Read the model definition and answer for the solid it produces. Units are mm, in the model's axes. Face numbers are marked on the shaded views. Coordinates: 2 decimals unless noted, no trailing zeros. Write each loop counter-clockwise with the first axis right and the second up, starting at its lowest first coordinate (ties: lowest second). Pieces come first, ordered by that corner, then holes. Notation, with made-up numbers: (86, 58) -> (111, 58) arc R27 cw to (111, 74) -> close; hole circle Ø6 at (61.25, -39.5). An arc over 180 degrees is marked (long way). One line per item, written item: value. Start each with the question number.
from build123d import *

# Parameters (mm, degrees)
ESQUISSE1_W         = 41
ESQUISSE1_H         = 30.4
BOSS_EXTRU_1_DEPTH  = 2
ESQUISSE3_R         = 3
BOSS_EXTRU_2_DEPTH  = 2
ESQUISSE4_W         = 15
ESQUISSE4_H         = 15.4
BOSS_EXTRU_3_DEPTH  = 2.5
BOSS_EXTRU_9_DEPTH  = 45
BOSS_EXTRU_10_DEPTH = 15
ESQUISSE13_W        = 2.172512758
ESQUISSE13_H        = 5.56
BOSS_EXTRU_11_DEPTH = 45
CONG_2_R            = 5
CONG_3_R            = 5
CONG_4_R            = 5


with BuildPart() as part:
    # Esquisse1 → Boss.-Extru.1 (new body)
    with BuildSketch(Plane(origin=(0, 0, 0), x_dir=(0, 0, -1), z_dir=(1, 0, 0))):
        with Locations((0, -15.2)):
            Rectangle(ESQUISSE1_W, ESQUISSE1_H)
    extrude(amount=BOSS_EXTRU_1_DEPTH)

    # Esquisse3 → Boss.-Extru.2 (add)
    with BuildSketch(Plane.XY.offset(20.5)):
        with BuildLine():
            Line((0, 0), (0, -30.4))
            Line((0, -30.4), (10, -30.4))
            ThreePointArc((10, -30.4), (12.121320344, -29.521320344), (13, -27.4))
            Line((13, -27.4), (13, -25.203998005))
            ThreePointArc((13, -25.203998005), (11.799859401, -22.431518929), (8.989283799, -21.323528643))
            ThreePointArc((8.989283799, -21.323528643), (7.793527962, -20.98117775), (6.868390743, -20.149819053))
            Line((6.868390743, -20.149819053), (6.868390743, -10.250180947))
            ThreePointArc((6.868390743, -10.250180947), (7.793527962, -9.41882225), (8.989283799, -9.076471357))
            ThreePointArc((8.989283799, -9.076471357), (11.799859401, -7.968481071), (13, -5.196001995))
            Line((13, -5.196001995), (13, -3))
            ThreePointArc((13, -3), (12.121320344, -0.878679656), (10, 0))
            Line((10, 0), (0, 0))
        make_face()
        with Locations((9, -4.61)):
            Circle(ESQUISSE3_R, mode=Mode.SUBTRACT)
        with Locations(Location((9, -25.79, 0), (0, 0, 180))):
            Circle(ESQUISSE3_R, mode=Mode.SUBTRACT)
    boss_extru_2 = extrude(amount=BOSS_EXTRU_2_DEPTH)

    # Symétrie1: Boss.-Extru.2 across plane
    add(boss_extru_2.mirror(Plane.XY))

    # Esquisse4 → Boss.-Extru.3 (add)
    with BuildSketch(Plane.ZY):
        with Locations((0, -15.2)):
            Rectangle(ESQUISSE4_W, ESQUISSE4_H)
    extrude(amount=BOSS_EXTRU_3_DEPTH)



with BuildPart() as body_2:
    # Esquisse11 → Boss.-Extru.9 (new body)
    with BuildSketch(Plane(origin=(0, 0, -22.5), x_dir=(-1, 0, 0), z_dir=(0, 0, -1))):
        Polygon((100, -86.630943166), (100, -89.130943166), (0, -35.96), (0, -33.46), align=None)
    extrude(amount=-BOSS_EXTRU_9_DEPTH)


with BuildPart() as part_1:
    add(part.part)

    add(body_2.part)  # Boss.-Extru.10 merges body 2
    # Esquisse12 → Boss.-Extru.10 (add)
    with BuildSketch(Plane(origin=(0, 0, -7.5), x_dir=(-1, 0, 0), z_dir=(0, 0, -1))):
        Polygon((2.5, -22.9), (20.844614881, -44.543278331), (25.445497181, -46.989610844), (2.5, -20.4), align=None)
    extrude(amount=-BOSS_EXTRU_10_DEPTH)

    # Esquisse13 → Boss.-Extru.11 (add)
    with BuildSketch(Plane(origin=(0, 0, -22.5), x_dir=(-1, 0, 0), z_dir=(0, 0, -1))):
        with Locations((-1.086256379, -33.18)):
            Rectangle(ESQUISSE13_W, ESQUISSE13_H)
    extrude(amount=-BOSS_EXTRU_11_DEPTH)

    # Congé2
    # the kernel refuses this fillet: 5 mm, written as the material it takes off along each edge
    with BuildSketch(Plane(origin=(2.172512758, -35.96, -32.809375556), x_dir=(0, 1, 0), z_dir=(0, 0, 1))) as cong_2_piece_1:
        with BuildLine():
            CenterArc((4.123750222, 5), CONG_2_R, 214.436842146, 55.563157854)
            Line((0, 2.172512758), (-0.082475004, 2.115963013))
            ThreePointArc((-0.082475004, 2.115963013), (-0.1, 1.086256379), (-0.1, 0))
            Line((-0.1, 0), (0, -0.1))
            Line((0, -0.1), (4.123750222, -0.1))
            Line((4.123750222, -0.1), (4.123750222, 0))
        make_face()
    extrude(amount=65.618751112, mode=Mode.SUBTRACT)

    # Congé3
    cong_3_edges = [part_1.edges().sort_by_distance(p)[0] for p in [
        (0, -33.46, 0),
    ]]
    fillet(cong_3_edges, radius=CONG_3_R)

    # Congé4
    # the kernel refuses this fillet: 5 mm, written as the material it adds along each edge
    with BuildSketch(Plane(origin=(-2.5, -20.4, -7.5), x_dir=(-0.6533220619728018, -0.7570801036479604, 0), z_dir=(0, 0, 1))) as cong_4_piece_1:
        with BuildLine():
            CenterArc((CONG_4_R * 0.3718225826, -CONG_4_R), CONG_4_R, 90, 40.792541927)
            Line((-CONG_4_R * 0.281499479373, -CONG_4_R * 0.242919896352), (0, 0))
            Line((0, 0), (CONG_4_R * 0.3718225826, 0))
        make_face()
    extrude(amount=15)
    # the kernel refuses this fillet: 5 mm, written as the material it takes off along each edge
    with BuildSketch(Plane(origin=(-2.5, -7.5, -18.325317547), x_dir=(1, 0, 0), z_dir=(0, 0, 1))) as cong_4_2_piece_1:
        with BuildLine():
            CenterArc((5, -4.330127019), CONG_4_R, 120, 60)
            Line((0, -4.330127019), (0, 0))
            Line((0, 0), (2.5, 0))
        make_face()
    extrude(amount=36.650635095, mode=Mode.SUBTRACT)


solid = part_1.part
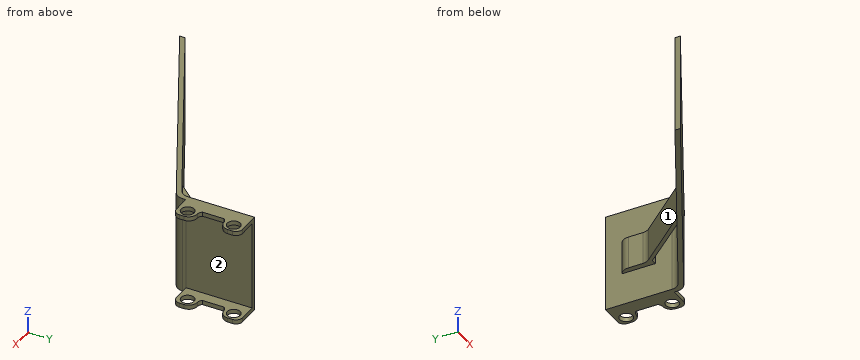
1. For a pull along Z with two mould halves and no side action, classify the marked faces 1 and 2 as +Z half, -Z half, draft (parallel to the pull), parting line (faces both ways), or undercut.
2. Given pin 1 (6 mm diameter, centred on y = -16, z = -12.5, fed in from -X); pin 2 (3 mm diameter, centred on y = -53, z = 16, fed in from +X); pin 3 (0.6 mm diameter, centred on y = -17, z = 21, fed in from +X); pin 4 (9.5 mm diameter, centred on x = 9, y = -25.79, fed in from +Z), each flat-ended and moving along its own axis, determine where each tip first touches the part or whether it passes through.
3. A cutting plane is placed at A-A on z = -1. Give the vertices of the cut face in (x, y), then the cut area to 3 significant figures.
4. Find the intervals of material crossed by probe 1 along Y at (x, z) = (9, -21); probe 2 along X at (y, z) = (-25.79, -21.05); probe 3 along X at (y, z) = (-3.5, -20), in increasing order. Write a range as from..to.
5. A cutting plane is placed at C-C on y = -50.5. Give the vertices of the cut face in (x, z).
6. A cutting plane is placed at B-B on x = -40. Give the vertices of the cut face in (y, z).
Derived:
1. face 1: draft
1. face 2: undercut
2. pin 1: stops at x = 0
2. pin 2: stops at x = -29.23
2. pin 3: stops at x = 6.87
2. pin 4: stops at z = 22.5
3. outline: (-100, -89.13) -> (0, -35.96) arc R5 ccw to (2.17, -31.84) -> (2.17, -30.4) -> (2, -30.4) -> (2, 0) -> (0, 0) -> (0, -7.5) arc R5 ccw to (-2.5, -11.83) -> (-2.5, -18.54) arc R5 cw to (-3.71, -21.81) -> (-25.45, -46.99) -> (-100, -86.63) -> close; hole (-20.84, -44.54) -> (-2.65, -34.87) arc R5 ccw to (0, -30.46) -> (0, -22.9) -> (-2.5, -22.9) -> close
3. area: 413 mm2
4. probe 1: y = -30.4..-28.79, -22.79..-21.32, -9.08..-7.61, -1.61..0
4. probe 2: x = 0..6, 12..13
4. probe 3: x = 0..2
5. outline: (-32.05, -22.5) -> (-27.35, -22.5) -> (-27.35, 22.5) -> (-32.05, 22.5) -> close
6. outline: (-57.23, -22.5) -> (-54.73, -22.5) -> (-54.73, 22.5) -> (-57.23, 22.5) -> close
